Input: part model. Units: mm. Frame: model coordinates. A direction names the side the tool comes from. Round coordinates to 2 decimals unless told otherwise and drop trailing zeros. Write each loop counter-clockwise with the first axis right and the second up, starting at its lowest first coordinate (ties: lowest second). Pieces come first, ordered by that corner, then holes. Notation, with made-up numbers: (-28, 81.25) - (-17, 81.25) arc R20 ccw to (-17, 93.25) - close; hole circle Ø2 at (-25, 47). An arc over 180 degrees is marked (long way). One line per item, written item: value. Start each with the question number.
```python
from build123d import *

# Parameters (mm, degrees)
SKETCH1_W               = 18.288
SKETCH1_H               = 63.35702232
SKETCH1_W_2             = 10.16
SKETCH1_H_2             = 5.08
BOSS_EXTRUDE1_DEPTH     = 12.7
BOSS_EXTRUDE2_DEPTH     = 18.288
CUT_EXTRUDE1_DEPTH      = 69.159320254
CUT_EXTRUDE1_DEPTH_BACK = 3.81
SKETCH6_R               = 2.159
CUT_EXTRUDE2_DEPTH      = 69.159320254
CUT_EXTRUDE2_DEPTH_BACK = 3.81
SKETCH9_R               = 2.159
CUT_EXTRUDE3_DEPTH      = 59.834546347
CUT_EXTRUDE3_DEPTH_BACK = 59.834546347
SKETCH10_R              = 1.778


with BuildPart() as part:
    # Sketch1 → Boss-Extrude1 (new body)
    with BuildSketch(Plane(origin=(0, 0, 0), x_dir=(1, 0, 0), z_dir=(0, 1, 0))):
        with Locations((9.144, 31.67851116)):
            Rectangle(SKETCH1_W, SKETCH1_H)
        with Locations((7.874, 55.73702232)):
            Rectangle(SKETCH1_W_2, SKETCH1_H_2, mode=Mode.SUBTRACT)
        with Locations((7.874, 7.62)):
            Rectangle(SKETCH1_W_2, SKETCH1_H_2, mode=Mode.SUBTRACT)
    extrude(amount=BOSS_EXTRUDE1_DEPTH)

    # Sketch2 → Boss-Extrude2 (add)
    with BuildSketch(Plane(origin=(18.288, 0, 0), x_dir=(0, 0, -1), z_dir=(1, 0, 0))):
        with BuildLine():
            Line((0, 12.7), (63.35702232, 12.7))
            ThreePointArc((63.35702232, 12.7), (31.67851116, 17.237450977), (0, 12.7))
        make_face()
    extrude(amount=-BOSS_EXTRUDE2_DEPTH)

    # Sketch6 → Cut-Extrude1 (cut, two sides: drawn at the far end of the back side and taken through both)
    with BuildSketch(Plane.XY.offset(-CUT_EXTRUDE1_DEPTH_BACK)):
        with Locations(Location((7.874, 6.35, 0), (0, 0, 180))):
            Circle(SKETCH6_R)
    extrude(amount=CUT_EXTRUDE1_DEPTH + CUT_EXTRUDE1_DEPTH_BACK, mode=Mode.SUBTRACT)

    # Sketch9 → Cut-Extrude2 (cut, two sides: drawn at the far end of the back side and taken through both)
    with BuildSketch(Plane(origin=(0, 0, -63.35702232), x_dir=(-1, 0, 0), z_dir=(0, 0, -1)).offset(-CUT_EXTRUDE2_DEPTH_BACK)):
        with Locations(Location((-8.128, 6.35, 0), (0, 0, 180))):
            Circle(SKETCH9_R)
    extrude(amount=CUT_EXTRUDE2_DEPTH + CUT_EXTRUDE2_DEPTH_BACK, mode=Mode.SUBTRACT)

    # Sketch10 → Cut-Extrude3 (cut, two sides: drawn at the far end of the back side and taken through both)
    with BuildSketch(Plane(origin=(0, 0, -53.19702232), x_dir=(-1, 0, 0), z_dir=(0, 0, -1)).offset(-CUT_EXTRUDE3_DEPTH_BACK)):
        with Locations((-8.128, 6.35)):
            Circle(SKETCH10_R)
    extrude(amount=CUT_EXTRUDE3_DEPTH + CUT_EXTRUDE3_DEPTH_BACK, mode=Mode.SUBTRACT)


solid = part.part
```
Q1. Access query for faces 4 (the flat face through (8, 12.7, -8)), 5 (the cylindrical face through (6.41, 7.66, -61.43)), 6 (the cylindrical face through (6.878, 8.265, -1.932)). Directions: +Z, -Z, +X, -X, +Y, -Y. A direction counts if a zero-diameter tool reaches every point of the face in a straight line with its end or side. Return the directions, or none.
Q2. Cut plane B-B, the plane x = 11.5. Output: boundary loops of the cut face in (y, z).
Q3. Cut plane D-D, the plane z = -14. Output: boundary loops of the cut face in (x, y).
Q4. Pull-direction query (Y, two-part tool) for faces 1 (the flat face through (12.954, 6, -56)), 2 (the flat face through (8, 12.7, -56)), 3 (the flat face through (6, 6, -3.81)); classes: pulls with the +Y half, pulls with the -Y half, needs draft (parallel to the pull), parting line crosses it, or undercut.
Q5. Contact query for flat-ended pins moving along their axis: pin 1 Ø1.3 at (x, y) = (8, 6.5) entering from -Z; pin 2 Ø4 at (x, y) = (8.128, 6.35) entering from -Z; pin 3 Ø3 at (x, z) = (10.5, -18) entering from +Y; pin 4 Ø4 at (y, z) = (4.5, -8.5) entering from -X. Output: stop coordinate, or through.
Q6. Cut plane C-C, the plane y = 11.5. Output: boundary loops of the cut face in (x, z).
Q7. Material intervals for probe 1 along Z at (x, y) = (12.75, 12); probe 2 along X at (y, z) = (6.35, -0.95) (3 decimals); probe 3 along X at (y, z) = (6.35, -4.6), sorted ascending. Write a range as from..to.
A:
1. face 4: -Y
1. face 5: -Z
1. face 6: +Z
2. outline: (0, -63.36) - (12.7, -63.36) arc R112.85 ccw to (12.7, 0) - (0, 0) - (0, -5.08) - (12.7, -5.08) - (12.7, -10.16) - (0, -10.16) - (0, -53.2) - (12.7, -53.2) - (12.7, -58.28) - (0, -58.28) - close
3. outline: (0, 0) - (18.29, 0) - (18.29, 15.84) - (0, 15.84) - close; hole circle Ø3.56 at (8.13, 6.35)
4. face 1: needs draft
4. face 2: pulls with the -Y half
4. face 3: undercut
5. pin 1: passes through
5. pin 2: stops at z = -59.55
5. pin 3: stops at y = 16.58
5. pin 4: stops at x = 0
6. outline: (0, -63.36) - (18.29, -63.36) - (18.29, 0) - (0, 0) - close; hole (2.79, -58.28) - (12.95, -58.28) - (12.95, -53.2) - (2.79, -53.2) - close; hole (2.79, -10.16) - (12.95, -10.16) - (12.95, -5.08) - (2.79, -5.08) - close
7. probe 1: z = -63.36..-58.28, -53.2..-10.16, -5.08..0
7. probe 2: x = 0..5.715, 10.033..18.288
7. probe 3: x = 0..6.35, 9.91..18.29
